Can you work these out from the model? Positions are in its coordinate system, mm. Round coordinates to 2 decimals unless told otherwise and drop trailing zeros. Write each loop counter-clockwise with the first axis right and the second up, starting at its lowest first coordinate (ties: lowest second). Pieces come first, ordered by that corner, then holes. Notation, with made-up numbers: (-2, 88.25) - (33, 88.25) arc R23 ccw to (33, 111.25) - close; hole circle Ø1 at (-32.5, 48.25). An arc over 180 degrees is marked (long way). One line per item, written item: value. Start each with the question number.
(1) I want a section at A-A on x = 0. List the corners of the cut face in (y, z) for me.
(2) If I drill on L1, parallel to Z at x = -22.5, y = 1.7; L2, parallel to X at y = 1.9, z = 4, over which ranges is the centre line in solid material (lowest first)? Write a range as from..to.
(3) I want a section at B-B on z = 0. List the corners of the cut face in (x, y) for me.
(4) I'm going to push flat-ended pins straight in: pin 1 Ø5 at (x, z) = (-22.5, -22.5) entering from +Y; pin 2 Ø1.5 at (y, z) = (1.5, 25.5) entering from -X; pin 3 Ø1 at (x, y) = (-33, 1) entering from +Z; pin 4 Ø1.5 at (y, z) = (0.5, -5.5) entering from -X. Where does each tip first touch, or does it pass through?
(5) I want a section at C-C on y = 2.1. Give the number of separate pieces and of enclosed holes in the cut face, plus the area to 3 significant figures.
(6) I want a section at D-D on x = -27. List the corners of the cut face in (y, z) for me, plus the area to 4 significant figures.
from build123d import *

# Parameters (mm, degrees)
SKETCH1_R           = 55
BOSS_EXTRUDE1_DEPTH = 3
SKETCH2_R           = 3
SKETCH2_W           = 25
SKETCH2_H           = 25
SKETCH2_W_2         = 3
SKETCH2_H_2         = 14
SKETCH2_W_3         = 14
SKETCH2_H_3         = 3
SKETCH2_H_4         = 7
CUT_EXTRUDE1_DEPTH  = 3


with BuildPart() as part:
    # Sketch1 → Boss-Extrude1 (new body)
    with BuildSketch(Plane(origin=(0, 0, 0), x_dir=(1, 0, 0), z_dir=(0, 1, 0))):
        Circle(SKETCH1_R)
    extrude(amount=BOSS_EXTRUDE1_DEPTH)

    # Sketch2 → Cut-Extrude1 (cut)
    with BuildSketch(Plane(origin=(0, 3, 0), x_dir=(1, 0, 0), z_dir=(0, 1, 0))):
        with Locations((-22.5, 22.5)):
            Circle(SKETCH2_R)
        with Locations((22.5, 22.5)):
            Circle(SKETCH2_R)
        with Locations((22.5, -22.5)):
            Circle(SKETCH2_R)
        with Locations((-22.5, -22.5)):
            Circle(SKETCH2_R)
        Rectangle(SKETCH2_W, SKETCH2_H)
        with Locations((0, 27.5)):
            Rectangle(SKETCH2_W_2, SKETCH2_H_2)
        with Locations((-27.5, 0)):
            Rectangle(SKETCH2_W_3, SKETCH2_H_3)
        with Locations((27.5, 0)):
            Rectangle(SKETCH2_W_3, SKETCH2_H_3)
        with Locations((0, -24)):
            Rectangle(SKETCH2_W_2, SKETCH2_H_4)
    extrude(amount=-CUT_EXTRUDE1_DEPTH, mode=Mode.SUBTRACT)


solid = part.part
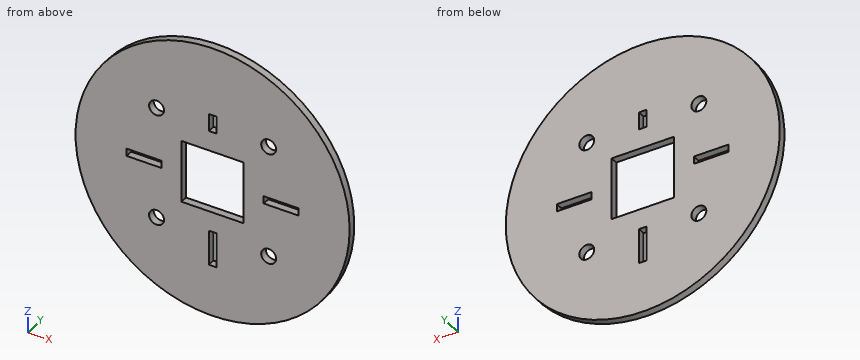
Established:
1. outline: (0, -55) - (3, -55) - (3, -34.5) - (0, -34.5) - close; (0, -20.5) - (3, -20.5) - (3, -12.5) - (0, -12.5) - close; (0, 12.5) - (3, 12.5) - (3, 20.5) - (0, 20.5) - close; (0, 27.5) - (3, 27.5) - (3, 55) - (0, 55) - close
2. L1: -50.19..-25.5, -19.5..-1.5, 1.5..19.5, 25.5..50.19
2. L2: -54.85..-12.5, 12.5..54.85
3. outline: (-55, 0) - (-34.5, 0) - (-34.5, 3) - (-55, 3) - close; (-20.5, 0) - (-12.5, 0) - (-12.5, 3) - (-20.5, 3) - close; (12.5, 0) - (20.5, 0) - (20.5, 3) - (12.5, 3) - close; (34.5, 0) - (55, 0) - (55, 3) - (34.5, 3) - close
4. pin 1: through
4. pin 2: x = -49.12
4. pin 3: z = 44.37
4. pin 4: x = -54.79
5. separate pieces: 1
5. enclosed holes: 9
5. area: 8,620 mm2
6. outline: (0, -47.92) - (3, -47.92) - (3, -1.5) - (0, -1.5) - close; (0, 1.5) - (3, 1.5) - (3, 47.92) - (0, 47.92) - close
6. area: 278.5 mm2
